Model file for the job. Use its own axes, mm. A direction names the side the tool comes from. Coordinates: 2 decimals unless noted, no trailing zeros. Write each loop counter-clockwise with the first axis right and the second up, starting at its lowest first coordinate (ties: lowest second). Pieces come first, ordered by that corner, then holes. Notation, with made-up numbers: (-19.75, 41.25) - (7.25, 41.25) arc R15 cw to (7.25, 53.25) - close; hole circle Ø8 at (10.25, 84). An arc over 180 degrees is marked (long way). Put each result on its own line as item: value. Start each with the question number.
1. Which spindle directions (+Z, -Z, +X, -X, +Y, -Y) get a long thin tool onto all of the face, cutting with end or side? Do faces 4 (the face through (56.077, 1.493, 45.777)), 5 (the face through (52.851, 1.458, 65.563)). Say none if no direction does.
2. Saw through at B-B, the plane z = 63.56. Write the cut outline in (x, y).
3. Pull direction X, two halves, no side cores. Call faces 1 (the face through (71.16, 0.99, 22.89)), 2 (the face through (0.45, 0.99, 1.43)), 3 (the face through (-3, 1, 48)): released by +X, released by -X, zero draft, split by the parting line, or undercut.
4. Saw through at D-D, the plane y = 0.55. Give the number of separate pieces and of enclosed holes in the cut face, plus the area to 4 significant figures.
5. Saw through at A-A, the plane x = 0. Write the cut outline in (y, z).
6. Drill centre lines: L1, parallel to Z at x = 61, y = 0.75; L2, parallel to Z at x = 24.5, y = 0.8; L3, parallel to X at y = 0.2, z = 27.5. Where is each one in solid material? Low to high. Write a range as from..to.
7. Drop flat-ended pins along their axis: P1, Ø4.5, axis at x = 56, z = 47.525, coming from the -Y side; P2, Ø2.5, axis at x = 52.22, z = 31.49, coming from the +Y side. Give the stop position or say it passes through.
8. Saw through at C-C, the plane x = 56. Write the cut outline in (y, z) (3 decimals).
```python
from build123d import *

# Parameters (mm, degrees)
CROQUIS1_R              = 1.8
CROQUIS1_R_2            = 1.5
CROQUIS1_R_3            = 1.75
SALIENTE_EXTRUIR1_DEPTH = 2
CROQUIS2_R              = 2.6
CORTAR_EXTRUIR1_DEPTH   = 1
CORTAR_EXTRUIR1_DRAFT   = -40
CROQUIS3_R              = 2.1
CORTAR_EXTRUIR2_DEPTH   = 1.1


with BuildPart() as part:
    # Croquis1 → Saliente-Extruir1 (new body)
    with BuildSketch(Plane(origin=(0, 0, 0), x_dir=(1, 0, 0), z_dir=(0, 1, 0))):
        with BuildLine():
            Line((1.012419451, 2.824005463), (69.732419451, -21.812442877))
            ThreePointArc((69.732419451, -21.812442877), (71.173289461, -22.909783687), (71.72, -24.63644834))
            Line((71.72, -24.63644834), (71.72, -70.41355166))
            ThreePointArc((71.72, -70.41355166), (71.173289461, -72.140216313), (69.732419451, -73.237557123))
            Line((69.732419451, -73.237557123), (1.012419451, -97.874005463))
            ThreePointArc((1.012419451, -97.874005463), (-1.726664653, -97.503289461), (-3, -95.05))
            Line((-3, -95.05), (-3, 0))
            ThreePointArc((-3, 0), (-1.726664653, 2.453289461), (1.012419451, 2.824005463))
        make_face()
        with Locations(Location((20, -26.675, 0), (0, 0, 270))):
            Circle(CROQUIS1_R, mode=Mode.SUBTRACT)
        with Locations(Location((20, -68.395, 0), (0, 0, 270))):
            Circle(CROQUIS1_R, mode=Mode.SUBTRACT)
        with Locations(Location((61.72, -26.675, 0), (0, 0, 270))):
            Circle(CROQUIS1_R, mode=Mode.SUBTRACT)
        with Locations(Location((61.72, -68.395, 0), (0, 0, 270))):
            Circle(CROQUIS1_R, mode=Mode.SUBTRACT)
        with Locations(Location((0, 0, 0), (0, 0, 270))):
            Circle(CROQUIS1_R_2, mode=Mode.SUBTRACT)
        with Locations(Location((0, -95.05, 0), (0, 0, 270))):
            Circle(CROQUIS1_R_2, mode=Mode.SUBTRACT)
        with Locations(Location((52.22, -31.49, 0), (0, 0, 270))):
            Circle(CROQUIS1_R_2, mode=Mode.SUBTRACT)
        with Locations(Location((52.22, -63.56, 0), (0, 0, 270))):
            Circle(CROQUIS1_R_2, mode=Mode.SUBTRACT)
        with Locations(Location((24, -70.925, 0), (0, 0, 270))):
            Circle(CROQUIS1_R_3, mode=Mode.SUBTRACT)
        with Locations(Location((24, -24.125, 0), (0, 0, 270))):
            Circle(CROQUIS1_R_3, mode=Mode.SUBTRACT)
        with Locations(Location((56, -47.525, 0), (0, 0, 270))):
            Circle(CROQUIS1_R_3, mode=Mode.SUBTRACT)
    extrude(amount=SALIENTE_EXTRUIR1_DEPTH)


with BuildPart() as cortar_extruir1_tool:
    # Croquis2 → Cortar-Extruir1 (with draft: the straight prism first)
    with BuildSketch(Plane.XZ):
        with Locations((56, 47.525)):
            Circle(CROQUIS2_R)
    extrude(amount=-CORTAR_EXTRUIR1_DEPTH)
    # Cortar-Extruir1: the draft: its side faces are tilted about the plane it starts from
    cortar_extruir1_sides = [cortar_extruir1_tool.faces().sort_by_distance(p)[0] for p in [
        (53.4, 0.5, 47.525),
    ]]
    draft(cortar_extruir1_sides, Plane.XZ, CORTAR_EXTRUIR1_DRAFT)


with BuildPart() as part_1:
    add(part.part)

    # Cortar-Extruir1: cut by cortar_extruir1_tool
    add(cortar_extruir1_tool.part, mode=Mode.SUBTRACT)

    # Croquis3 → Cortar-Extruir2 (cut)
    with BuildSketch(Plane(origin=(0, 2, 0), x_dir=(1, 0, 0), z_dir=(0, 1, 0))):
        with Locations(Location((52.22, -31.49, 0), (0, 0, 270))):
            Circle(CROQUIS3_R)
        with Locations(Location((52.22, -63.56, 0), (0, 0, 270))):
            Circle(CROQUIS3_R)
    extrude(amount=-CORTAR_EXTRUIR2_DEPTH, mode=Mode.SUBTRACT)


solid = part_1.part
```
Final values:
1. face 4: +Y, -Y
1. face 5: +Y
2. outline: (-3, 0) - (50.72, 0) - (50.72, 0.9) - (50.12, 0.9) - (50.12, 2) - (-3, 2) - close; (53.72, 0) - (71.72, 0) - (71.72, 2) - (54.32, 2) - (54.32, 0.9) - (53.72, 0.9) - close
3. face 1: released by +X
3. face 2: undercut
3. face 3: released by -X
4. separate pieces: 1
4. enclosed holes: 11
4. area: 5,625 mm²
5. outline: (0, -3) - (2, -3) - (2, -1.5) - (0, -1.5) - close; (0, 1.5) - (2, 1.5) - (2, 93.55) - (0, 93.55) - close; (0, 96.55) - (2, 96.55) - (2, 98.05) - (0, 98.05) - close
6. L1: z = 18.68..25.03, 28.32..66.75, 70.04..76.37
6. L2: z = 5.6..22.45, 25.8..69.25, 72.6..89.45
6. L3: x = -3..18.4, 21.6..60.12, 63.32..71.72
7. P1: stops at y = 0.42
7. P2: passes through
8. outline: (0, 16.889) - (2, 16.889) - (2, 45.775) - (1, 45.775) - (1, 45.764) - (0, 44.925) - close; (0, 50.125) - (1, 49.286) - (1, 49.275) - (2, 49.275) - (2, 78.161) - (0, 78.161) - close
